For this review, take the finished solid that the model builds, in its own axes (mm). A direction names the side the tool comes from. Coordinates: 2 decimals unless noted, no trailing zeros. Loops run counter-clockwise (first coordinate to the right, second up) from the corner with the lowest first, then second, coordinate; pieces in that order, holes last. Notation, with made-up numbers: M 58.25,70 L 75.25,70 A17 ccw 75.25,98 Z; hole C 71.25,-20.75 d8. An arc over 180 degrees is marked long. Answer as a JSON object with one key per item and string values. Group by question number.
Item 1: Add section D-D (z = 28). State the section outline as (x, y) points, then the cut area to 3 significant figures.
Item 2: Tool access review of faces 1 (the face through (37.58, 3.15, 8.89)), 2 (the face through (0, -15, 9)), 3 (the face through (-11.798, -10.348, 24.661)): name each direction out of +Z, -Z, +X, -X, +Y, -Y from which nothing blocks a thin tool from reaching the whole face with its end or side.
Item 3: Wall thickness on L1, parallel to Y at x = 27.9, z = 14; L2, parallel to Y at x = 27, z = 14; L3, parallel to Z at x = 12.5, y = -7.75: over which ranges is each line inside the solid? List them lowest first. Write a range as from..to.
Item 4: Insertion check: pin 1 (2 mm diameter, centred on x = 18, y = 8.5, fed in from -Z); pin 2 (2 mm diameter, centred on y = 6.5, z = 21, fed in from +X); pin 3 (2 mm diameter, centred on x = 30.5, y = 4.5, fed in from +Z); pin 4 (2 mm diameter, centred on y = 10.5, z = 7.5, fed in from +X). Each pin has a flat end and moves straight along its axis. Give the tip position at first contact, or say it passes through.
Item 5: Add section A-A (z = 13). State the section outline as (x, y) points, then the cut area to 3 significant figures.
Item 6: Add section B-B (x = -9.5). State the section outline as (y, z) points, then the cut area to 3 significant figures.
Item 7: Mouldability with a two-part tool opening along Y and no side actions: class faces 4 (the face through (26.3, -11.4, 9.3)), 5 (the face through (25.902, 10.288, 9.329)), 6 (the face through (0, 15, 9)), 7 (the face through (0, 0, 0)) as +Y half, -Y half, draft (parallel to the pull), parting line (faces both ways), or undercut.
Item 8: Add section C-C (y = 0). State the section outline as (x, z) points, then the cut area to 3 significant figures.
from build123d import *

# Parameters (mm, degrees)
ESQUISSE1_W             = 65
ESQUISSE1_H             = 30
BOSS_EXTRU_1_DEPTH      = 18.4
ESQUISSE2_R             = 10.6
BOSS_EXTRU_2_DEPTH      = 12.7
ESQUISSE4_R             = 2
ENL_V_MAT_EXTRU_2_DEPTH = 41.246863232
ESQUISSE5_R             = 2
ENL_V_MAT_EXTRU_3_DEPTH = 41.246863232
ESQUISSE6_R             = 5.18
BOSS_EXTRU_3_DEPTH      = 10.3


with BuildPart() as part:
    # Esquisse1 → Boss.-Extru.1 (new body)
    with BuildSketch(Plane.XY):
        Rectangle(ESQUISSE1_W, ESQUISSE1_H)
    extrude(amount=BOSS_EXTRU_1_DEPTH)

    # Esquisse2 → Boss.-Extru.2 (add)
    with BuildSketch(Plane.XY.offset(18.4)):
        with Locations((-9.5, 0)):
            Circle(ESQUISSE2_R)
    extrude(amount=BOSS_EXTRU_2_DEPTH)

    # Esquisse4 → Enlèv. mat.-Extru.2 (cut, through all)
    with BuildSketch(Plane.XY.offset(18.4)):
        with Locations((27.9, -10.2)):
            Circle(ESQUISSE4_R)
    extrude(amount=-ENL_V_MAT_EXTRU_2_DEPTH, mode=Mode.SUBTRACT)

    # Esquisse5 → Enlèv. mat.-Extru.3 (cut, through all)
    with BuildSketch(Plane.XY.offset(18.4)):
        with Locations((27.9, 10.2)):
            Circle(ESQUISSE5_R)
    extrude(amount=-ENL_V_MAT_EXTRU_3_DEPTH, mode=Mode.SUBTRACT)

    # Esquisse6 → Boss.-Extru.3 (add)
    with BuildSketch(Plane(origin=(32.5, 0, 0), x_dir=(0, 0, -1), z_dir=(1, 0, 0))):
        with Locations(Location((-13, 0, 0), (0, 0, 180))):
            Circle(ESQUISSE6_R)
    extrude(amount=BOSS_EXTRU_3_DEPTH)


solid = part.part
From the geometry:
{
 "1": {"outline": "C -9.5,0 d21.2", "area": "353 mm²"},
 "2": {"face 1": "+X", "face 2": "+Z, -Z, +X, -X, -Y", "face 3": "+Z"},
 "3": {"L1": "y = -15..-12.2, -8.2..8.2, 12.2..15", "L2": "y = -15..-11.99, -8.41..8.41, 11.99..15", "L3": "z = 0..18.4"},
 "4": {"pin 1": "stops at z = 0", "pin 2": "stops at x = -0.44", "pin 3": "stops at z = 18.4", "pin 4": "stops at x = 32.5"},
 "5": {"outline": "M -32.5,-15 L 32.5,-15 L 32.5,-5.18 L 42.8,-5.18 L 42.8,5.18 L 32.5,5.18 L 32.5,15 L -32.5,15 Z; hole C 27.9,-10.2 d4; hole C 27.9,10.2 d4", "area": "2,030 mm²"},
 "6": {"outline": "M -15,0 L 15,0 L 15,18.4 L 10.6,18.4 L 10.6,31.1 L -10.6,31.1 L -10.6,18.4 L -15,18.4 Z", "area": "821 mm²"},
 "7": {"face 4": "undercut", "face 5": "undercut", "face 6": "+Y half", "face 7": "draft"},
 "8": {"outline": "M -32.5,0 L 32.5,0 L 32.5,7.82 L 42.8,7.82 L 42.8,18.18 L 32.5,18.18 L 32.5,18.4 L 1.1,18.4 L 1.1,31.1 L -20.1,31.1 L -20.1,18.4 L -32.5,18.4 Z", "area": "1,570 mm²"}
}
